Build history of the part. All positions in model axes, mm. A direction names the side the tool comes from. Round coordinates to 2 decimals unless told otherwise and drop trailing zeros. Loops run counter-clockwise (first coordinate to the right, second up) from the corner with the lowest first, then second, coordinate; pieces in that order, holes last. Notation, with made-up numbers: (52.5, -15.5) - (78.5, -15.5) arc R9 cw to (78.5, -5.5) - close; hole circle Ø6 at (-8.75, 5.25). An arc over 180 degrees is marked (long way). Answer as CSV lines item,"result". Start each with the question number.
```python
from build123d import *

# Parameters (mm, degrees)
SKETCH1_W           = 304.8
SKETCH1_H           = 50.8
SKETCH1_R           = 2.4892
BOSS_EXTRUDE1_DEPTH = 6.35
SKETCH3_W           = 165.1
SKETCH3_H           = 25.4
CUT_EXTRUDE1_DEPTH  = 155.632604906
FILLET1_R           = 6.35


with BuildPart() as part:
    # Sketch1 → Boss-Extrude1 (new body)
    with BuildSketch(Plane.XY):
        Rectangle(SKETCH1_W, SKETCH1_H)
        with Locations((-88.9, 16.51)):
            Circle(SKETCH1_R, mode=Mode.SUBTRACT)
        with Locations((-88.9, -16.51)):
            Circle(SKETCH1_R, mode=Mode.SUBTRACT)
        with Locations((88.9, -16.51)):
            Circle(SKETCH1_R, mode=Mode.SUBTRACT)
        with Locations((88.9, 16.51)):
            Circle(SKETCH1_R, mode=Mode.SUBTRACT)
        with Locations((-147.828, 11.43)):
            Circle(SKETCH1_R, mode=Mode.SUBTRACT)
        with Locations((-147.828, -11.43)):
            Circle(SKETCH1_R, mode=Mode.SUBTRACT)
        with Locations((147.828, 11.43)):
            Circle(SKETCH1_R, mode=Mode.SUBTRACT)
        with Locations((147.828, -11.43)):
            Circle(SKETCH1_R, mode=Mode.SUBTRACT)
    extrude(amount=BOSS_EXTRUDE1_DEPTH)

    # Sketch3 → Cut-Extrude1 (cut, through all)
    with BuildSketch(Plane.XY.offset(6.35)):
        with Locations((0, -12.7)):
            Rectangle(SKETCH3_W, SKETCH3_H)
    extrude(amount=-CUT_EXTRUDE1_DEPTH, mode=Mode.SUBTRACT)

    # Fillet1
    fillet1_edges = [part.edges().sort_by_distance(p)[0] for p in [
        (-82.55, 0, 3.175),
        (82.55, 0, 3.175),
    ]]
    fillet(fillet1_edges, radius=FILLET1_R)


solid = part.part
```
Q1. Tool access for faces 4 (the cylindrical face through (-80.74, -1.91, 3.13)), 5 (the cylindrical face through (86.413, -16.401, 3.131)): list every direction of +Z, -Z, +X, -X, +Y, -Y with a clear straight run to the whole face (end or side of a thin tool).
Q2. Two-plate mould, pull along X, no slides. Class faces 1 (the cylindrical face through (-146.49, 13.53, 3.13)), 2 (the flat face through (-152.4, 0, 3)), 3 (the flat face through (-118, -25.4, 3)): released by +X, released by -X, zero draft, split by the parting line, or undercut.
Q3. Wall check: probe 1 along X at (y, z) = (16, 0.5); probe 2 along Y at (x, z) = (88.9, 3); probe 3 along X at (y, z) = (-20, 4.5). Give the ranges that are in metal, low to high. Write a range as [from, to].
Q4. Band-saw the part on B-B, the plane z = 3.25. Give the number of separate pieces and of enclosed holes in the cut face, then the cut area to 3 significant figures.
Q5. Pin check, flat tip, straight feed: pin 1 Ø3 at (x, z) = (62.5, 1.5) entering from -Y. Stop position of the tip, or through.
Q6. Band-saw the part on D-D, the plane y = 16.51. List the corners of the cut face in (x, z), then the cut area to 3 significant figures.
Q7. Band-saw the part on C-C, the plane x = -88.9. List the corners of the cut face in (y, z).
Q8. Band-saw the part on A-A, the plane y = -16.51. List the corners of the cut face in (x, z).
Reported:
1,face 4,"+Z, -Z, -Y"
1,face 5,"+Z, -Z"
2,face 1,"undercut"
2,face 2,"released by -X"
2,face 3,"zero draft"
3,probe 1,"x = [-152.4, -91.34], [-86.46, 86.46], [91.34, 152.4]"
3,probe 2,"y = [-25.4, -19], [-14.02, 14.02], [19, 25.4]"
3,probe 3,"x = [-152.4, -82.55], [82.55, 152.4]"
4,separate pieces,"1"
4,enclosed holes,"8"
4,area,"11,200 mm2"
5,pin 1,"stops at y = 0"
6,outline,"(-152.4, 0) - (-91.39, 0) - (-91.39, 6.35) - (-152.4, 6.35) - close; (-86.41, 0) - (86.41, 0) - (86.41, 6.35) - (-86.41, 6.35) - close; (91.39, 0) - (152.4, 0) - (152.4, 6.35) - (91.39, 6.35) - close"
6,area,"1,870 mm2"
7,outline,"(-25.4, 0) - (-19, 0) - (-19, 6.35) - (-25.4, 6.35) - close; (-14.02, 0) - (14.02, 0) - (14.02, 6.35) - (-14.02, 6.35) - close; (19, 0) - (25.4, 0) - (25.4, 6.35) - (19, 6.35) - close"
8,outline,"(-152.4, 0) - (-91.39, 0) - (-91.39, 6.35) - (-152.4, 6.35) - close; (-86.41, 0) - (-82.55, 0) - (-82.55, 6.35) - (-86.41, 6.35) - close; (82.55, 0) - (86.41, 0) - (86.41, 6.35) - (82.55, 6.35) - close; (91.39, 0) - (152.4, 0) - (152.4, 6.35) - (91.39, 6.35) - close"
